from build123d import *

# Parameters (mm, degrees)
SKETCH1_W           = 100
SKETCH1_H           = 100
BOSS_EXTRUDE1_DEPTH = 2
SKETCH2_R           = 1.25
BOSS_EXTRUDE2_DEPTH = 20
FILLET1_R           = 1
FILLET2_R           = 5


with BuildPart() as part:
    # Sketch1 → Boss-Extrude1 (new body)
    with BuildSketch(Plane(origin=(0, 0, 0), x_dir=(1, 0, 0), z_dir=(0, 1, 0))):
        Rectangle(SKETCH1_W, SKETCH1_H)
    extrude(amount=BOSS_EXTRUDE1_DEPTH)

    # Sketch2 → Boss-Extrude2 (add)
    with BuildSketch(Plane(origin=(0, 0, 0), x_dir=(1, 0, 0), z_dir=(0, 1, 0))):
        with Locations(Location((-20, -20, 0), (0, 0, 270))):
            Circle(SKETCH2_R)
        with Locations(Location((-20, 20, 0), (0, 0, 270))):
            Circle(SKETCH2_R)
        with Locations(Location((20, 20, 0), (0, 0, 270))):
            Circle(SKETCH2_R)
        with Locations(Location((20, -20, 0), (0, 0, 270))):
            Circle(SKETCH2_R)
    extrude(amount=BOSS_EXTRUDE2_DEPTH)

    # Fillet1
    fillet1_edges = [part.edges().sort_by_distance(p)[0] for p in [
        (-50, 2, 0),
        (0, 2, 50),
        (50, 2, 0),
        (0, 2, -50),
    ]]
    fillet(fillet1_edges, radius=FILLET1_R)

    # Fillet2
    # the kernel refuses this fillet: 5 mm, written as the material it takes off along each edge
    with BuildSketch(Plane(origin=(-45, 2, 45), x_dir=(-1, 0, 0), z_dir=(0, 0, -1))) as fillet2_piece_1:
        with BuildLine():
            CenterArc((4, -1), 1, 0, 90)
            Line((5, -1), (5, 0))
            Line((5, 0), (4, 0))
        make_face()
    revolve(axis=Axis((-45, 2, 45), (0, 1, 0)), revolution_arc=90, mode=Mode.SUBTRACT)
    with BuildSketch(Plane(origin=(-45, 2, -45), x_dir=(0, 0, -1), z_dir=(1, 0, 0))) as fillet2_piece_2:
        with BuildLine():
            CenterArc((4, -1), 1, 0, 90)
            Line((5, -1), (5, 0))
            Line((5, 0), (4, 0))
        make_face()
    revolve(axis=Axis((-45, 2, -45), (0, 1, 0)), revolution_arc=90, mode=Mode.SUBTRACT)
    with BuildSketch(Plane(origin=(45, 2, 45), x_dir=(0, 0, 1), z_dir=(-1, 0, 0))) as fillet2_piece_3:
        with BuildLine():
            CenterArc((4, -1), 1, 0, 90)
            Line((5, -1), (5, 0))
            Line((5, 0), (4, 0))
        make_face()
    revolve(axis=Axis((45, 2, 45), (0, 1, 0)), revolution_arc=90, mode=Mode.SUBTRACT)
    with BuildSketch(Plane(origin=(45, 2, -45), x_dir=(1, 0, 0), z_dir=(0, 0, 1))) as fillet2_piece_4:
        with BuildLine():
            CenterArc((4, -1), 1, 0, 90)
            Line((5, -1), (5, 0))
            Line((5, 0), (4, 0))
        make_face()
    revolve(axis=Axis((45, 2, -45), (0, 1, 0)), revolution_arc=90, mode=Mode.SUBTRACT)
    with BuildSketch(Plane(origin=(50, -12.5, -50), x_dir=(-1, 0, 0), z_dir=(0, 1, 0)), Plane(origin=(50, -12.5, 50), x_dir=(0, 0, -1), z_dir=(0, 1, 0))) as fillet2_piece_5:
        with BuildLine():
            CenterArc((FILLET2_R, FILLET2_R), FILLET2_R, 180, 90)
            Line((0, FILLET2_R), (0, 0))
            Line((0, 0), (FILLET2_R, 0))
        make_face()
    extrude(amount=14.5, mode=Mode.SUBTRACT)
    with BuildSketch(Plane(origin=(-50, -12.5, -50), x_dir=(1, 0, 0), z_dir=(0, 1, 0)), Plane(origin=(-50, -12.5, 50), x_dir=(0, 0, -1), z_dir=(0, 1, 0))) as fillet2_piece_6:
        with BuildLine():
            CenterArc((FILLET2_R, -FILLET2_R), FILLET2_R, 90, 90)
            Line((0, -FILLET2_R), (0, 0))
            Line((0, 0), (FILLET2_R, 0))
        make_face()
    extrude(amount=14.5, mode=Mode.SUBTRACT)


solid = part.part
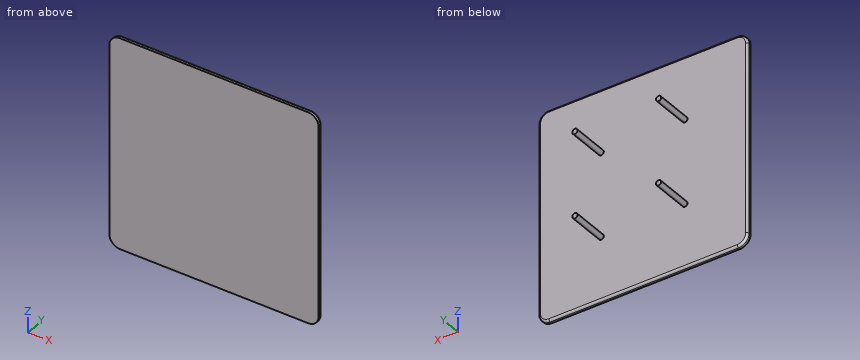
Part model, mm, in its own coordinate system. Coordinates: 2 decimals unless noted, no trailing zeros. Loops run counter-clockwise (first coordinate to the right, second up) from the corner with the lowest first, then second, coordinate; pieces in that order, holes last. Notation, with made-up numbers: (-40, 31.5) - (16, 31.5) arc R28 ccw to (16, 57.5) - close; hole circle Ø1 at (18.5, 23.5). An arc over 180 degrees is marked (long way). Write each question's results on one line, items separated by ' | '. Start each with the question number.
Q1. Slice it at C-C on z = 20. Give the cut face in (x, y).
Q2. Slice it at B-B on y = 15.5. Give the cut face in (x, z).
Q3. Slice it at D-D on z = -4. Give the cut face in (x, y), and give its area (3 significant figures).
Q4. Probe line 1 along Y through (x, z) = (-25, -32); line 2 along X through (y, z) = (1.5, 20). List the from-to ranges inside material, lowest first.
Q5. Drop flat-ended pins along their axis: pin 1 Ø4 at (x, z) = (29.5, -34.5) entering from +Y; pin 2 Ø1 at (y, z) = (3, 25.5) entering from -X; pin 3 Ø1 at (x, y) = (-21, 2) entering from +Z. Give the stop position or say it passes through.
Q6. Slice it at A-A on x = -20. Give the cut face in (y, z), and give its area (3 significant figures).
Answer:
1) outline: (-50, 0) - (50, 0) - (50, 1) arc R1 ccw to (49, 2) - (21.25, 2) - (21.25, 20) - (18.75, 20) - (18.75, 2) - (-18.75, 2) - (-18.75, 20) - (-21.25, 20) - (-21.25, 2) - (-49, 2) arc R1 ccw to (-50, 1) - close
2) outline: circle Ø2.5 at (-20, -20); circle Ø2.5 at (-20, 20); circle Ø2.5 at (20, -20); circle Ø2.5 at (20, 20)
3) outline: (-50, 0) - (50, 0) - (50, 1) arc R1 ccw to (49, 2) - (-49, 2) arc R1 ccw to (-50, 1) - close | area: 200 mm2
4) line 1: y = 0 to 2 | line 2: x = -49.87 to 49.87
5) pin 1: stops at y = 2 | pin 2: passes through | pin 3: stops at z = 49.87
6) outline: (0, -50) - (1, -50) arc R1 ccw to (2, -49) - (2, -21.25) - (20, -21.25) - (20, -18.75) - (2, -18.75) - (2, 18.75) - (20, 18.75) - (20, 21.25) - (2, 21.25) - (2, 49) arc R1 ccw to (1, 50) - (0, 50) - close | area: 290 mm2
